from build123d import *

# Parameters (mm, degrees)
RESSALTO_EXTRUS_O2_DEPTH   = 12.5
RESSALTO_EXTRUS_O2_2_DEPTH = 12.5
ESBO_O2_W                  = 7.5
ESBO_O2_H                  = 64.1
RESSALTO_EXTRUS_O3_DEPTH   = 28
ESBO_O3_W                  = 50
ESBO_O3_H                  = 90
RESSALTO_EXTRUS_O4_DEPTH   = 5
RESSALTO_EXTRUS_O5_DEPTH   = 28


with BuildPart() as part:
    # Esbo_o1 → Ressalto-extrus_o2 (new body)
    with BuildSketch(Plane.XY):
        with BuildLine():
            Line((-4.763139721, 2.75), (-8.569568251, 2.75))
            ThreePointArc((-8.569568251, 2.75), (-2.576160071, 8.623421553), (5.656854249, 7))
            Line((5.656854249, 7), (15.656854249, 7))
            Line((15.656854249, 7), (15.656854249, -7))
            Line((15.656854249, -7), (5.656854249, -7))
            ThreePointArc((5.656854249, -7), (-2.576160071, -8.623421553), (-8.569568251, -2.75))
            Line((-8.569568251, -2.75), (-4.763139721, -2.75))
            ThreePointArc((-4.763139721, -2.75), (5.5, 0), (-4.763139721, 2.75))
        make_face()
    ressalto_extrus_o2 = extrude(amount=RESSALTO_EXTRUS_O2_DEPTH)



with BuildPart() as body_2:
    # Esbo_o1 → Ressalto-extrus_o2 2 (new body)
    with BuildSketch(Plane.XY):
        with BuildLine():
            Line((15.656854249, -57.1), (15.656854249, -43.1))
            Line((15.656854249, -43.1), (5.656854249, -43.1))
            ThreePointArc((5.656854249, -43.1), (-2.576160071, -41.476578447), (-8.569568251, -47.35))
            Line((-8.569568251, -47.35), (-4.763139721, -47.35))
            ThreePointArc((-4.763139721, -47.35), (5.5, -50.1), (-4.763139721, -52.85))
            Line((-4.763139721, -52.85), (-8.569568251, -52.85))
            ThreePointArc((-8.569568251, -52.85), (-2.576160071, -58.723421553), (5.656854249, -57.1))
            Line((5.656854249, -57.1), (15.656854249, -57.1))
        make_face()
    ressalto_extrus_o2_2 = extrude(amount=RESSALTO_EXTRUS_O2_2_DEPTH)


with BuildPart() as part_1:
    add(part.part)

    add(body_2.part)  # Ressalto-extrus_o3 merges body 2
    # Esbo_o2 → Ressalto-extrus_o3 (add)
    with BuildSketch(Plane(origin=(0, 0, 12.5), x_dir=(-1, 0, 0), z_dir=(0, 0, -1))):
        with Locations((-11.906854249, -25.05)):
            Rectangle(ESBO_O2_W, ESBO_O2_H)
    ressalto_extrus_o3 = extrude(amount=RESSALTO_EXTRUS_O3_DEPTH)

    # Esbo_o3 → Ressalto-extrus_o4 (add)
    with BuildSketch(Plane(origin=(0, 0, -15.5), x_dir=(-1, 0, 0), z_dir=(0, 0, -1))):
        with Locations((9.343145751, -38)):
            Rectangle(ESBO_O3_W, ESBO_O3_H)
    ressalto_extrus_o4 = extrude(amount=RESSALTO_EXTRUS_O4_DEPTH)

    # Esbo_o4 → Ressalto-extrus_o5 (add)
    with BuildSketch(Plane.XY.offset(-15.5)):
        Polygon((15.656854249, -83), (-34.343145751, -83), (-34.343145751, -63), (8.156854249, -63), (8.156854249, -57.1), (15.656854249, -57.1), (15.656854249, -63), align=None)
    ressalto_extrus_o5 = extrude(amount=RESSALTO_EXTRUS_O5_DEPTH)

    # Espelhar4: Ressalto-extrus_o4, Ressalto-extrus_o5 across plane
    add(ressalto_extrus_o4.mirror(Plane(origin=(-34.343145751, 0, 0), x_dir=(0, 0, 1), z_dir=(1, 0, 0))))
    add(ressalto_extrus_o5.mirror(Plane(origin=(-34.343145751, 0, 0), x_dir=(0, 0, 1), z_dir=(1, 0, 0))))

    # Espelhar5: Ressalto-extrus_o3 across plane
    add(ressalto_extrus_o3.mirror(Plane(origin=(-34.343145751, 0, 0), x_dir=(0, 0, 1), z_dir=(1, 0, 0))))

    # Espelhar6: Ressalto-extrus_o2, Ressalto-extrus_o2 2 across plane
    add(ressalto_extrus_o2.mirror(Plane(origin=(-34.343145751, 0, 0), x_dir=(0, 0, 1), z_dir=(1, 0, 0))))
    add(ressalto_extrus_o2_2.mirror(Plane(origin=(-34.343145751, 0, 0), x_dir=(0, 0, 1), z_dir=(1, 0, 0))))


solid = part_1.part
The listing builds one solid part. Answer for the finished solid, in the listing's coordinates (mm). A direction names the side the tool comes from. Coordinates: 2 decimals unless noted, no trailing zeros. Loops run counter-clockwise (first coordinate to the right, second up) from the corner with the lowest first, then second, coordinate; pieces in that order, holes last. Notation, with made-up numbers: M 39.25,72 L 76.25,72 A18 ccw 76.25,81 Z; hole C 55.5,-40 d6. An arc over 180 degrees is marked long. Answer in a Markdown table with one row per item.
1) Find the intervals of material crossed by probe 1 along Y at (x, z) = (0, 9.75); probe 2 along X at (y, z) = (-50, 3); probe 3 along X at (y, z) = (-56, -4.5), in increasing order.
Answers below:
| item | result |
|---|---|
| probe 1 | -83 to -63, -59.1 to -55.6, -44.6 to -41.1, -9 to -5.5, 5.5 to 9 |
| probe 2 | -84.34 to -74.19, 5.5 to 15.66 |
| probe 3 | -84.34 to -76.84, 8.16 to 15.66 |
2) Determine the mould class of faces 1 (the cylindrical face through (-74.183, -0.202, 6.162)), 2 (the flat face through (-74, 2, 0)), 3 (the flat face through (-76.843, -28, -4)) for opening direction Z: released by +Z, released by -Z, zero draft, split by the parting line, or undercut.
Answers below:
| item | result |
|---|---|
| face 1 | zero draft |
| face 2 | undercut |
| face 3 | undercut |
3) Find section D-D (x = -28). Determine the outline of the cut face in (y, z).
Answers below:
| item | result |
|---|---|
| outline | M -83,-20.5 L 7,-20.5 L 7,-15.5 L -63,-15.5 L -63,12.5 L -83,12.5 Z |
4) Find section A-A (x = 0). Determine the outline of the cut face in (y, z), then the cut area to 4 significant figures.
Answers below:
| item | result |
|---|---|
| outline | M -83,-20.5 L 7,-20.5 L 7,-15.5 L -63,-15.5 L -63,12.5 L -83,12.5 Z; M -59.1,0 L -55.6,0 L -55.6,12.5 L -59.1,12.5 Z; M -44.6,0 L -41.1,0 L -41.1,12.5 L -44.6,12.5 Z; M -9,0 L -5.5,0 L -5.5,12.5 L -9,12.5 Z; M 5.5,0 L 9,0 L 9,12.5 L 5.5,12.5 Z |
| area | 1,185 mm^2 |
5) Given pin 1 (1.1 mm diameter, centred on x = -7, z = 5, fed in from +Y); pin 2 (3 mm diameter, centred on x = -75.5, z = 3.5, fed in from +Y); pin 3 (1.5 mm diameter, centred on x = -35.5, z = -16.5, fed in from +Y), each flat-ended and moving along its own axis, determine where each tip first touches the part or whether it passes through.
Answers below:
| item | result |
|---|---|
| pin 1 | y = 6.28 |
| pin 2 | y = 7.26 |
| pin 3 | y = 7 |
6) Which of the six approach directions +Z, -Z, +X, -X, +Y, -Y give full straight-line access (tool end or side, diameter ignored) to faces 4 (the flat face through (7, -7, 6)), 5 (the cylindrical face through (-2.69, 8.59, 6.16)), 6 (the flat face through (8.157, -28, -5)), 7 (the flat face through (15.657, -39, -4)), 8 (the flat face through (5.3, -48, 0))?
Answers below:
| item | result |
|---|---|
| face 4 | +Z |
| face 5 | +Z, +Y |
| face 6 | none |
| face 7 | +Z, -Z, +X, +Y, -Y |
| face 8 | +Y |
7) Find section B-B (y = -14). Determine the outline of the cut face in (x, z).
Answers below:
| item | result |
|---|---|
| outline | M -84.34,-20.5 L 15.66,-20.5 L 15.66,12.5 L 8.16,12.5 L 8.16,-15.5 L -76.84,-15.5 L -76.84,12.5 L -84.34,12.5 Z |
8) Find section C-C (z = -6). Determine the outline of the cut face in (x, y).
Answers below:
| item | result |
|---|---|
| outline | M -84.34,-83 L 15.66,-83 L 15.66,7 L 8.16,7 L 8.16,-63 L -76.84,-63 L -76.84,7 L -84.34,7 Z |
